Can you work these out from the model? Positions are in its coordinate system, mm. A direction names the side the tool comes from. Coordinates: 2 decimals unless noted, no trailing zeros. Write each loop counter-clockwise with the first axis right and the second up, starting at its lowest first coordinate (ties: lowest second). Pieces come first, ordered by that corner, then holes. Notation, with made-up numbers: (-37, 75) -> (-33, 75) arc R35 ccw to (-33, 108) -> close; hole circle Ø7 at (-14, -21). An arc over 180 degrees is marked (long way). Use one line per item in the form item = value.
```python
from build123d import *

# Parameters (mm, degrees)
SKETCH1_R           = 1.5
SKETCH1_W           = 4.5
SKETCH1_H           = 4.5
BOSS_EXTRUDE1_DEPTH = 2.5


with BuildPart() as part:
    # Sketch1 → Boss-Extrude1 (new body, symmetric)
    with BuildSketch(Plane(origin=(0, 0, 0), x_dir=(1, 0, 0), z_dir=(0, 1, 0))):
        with BuildLine():
            Line((-30, 50), (30, 50))
            ThreePointArc((30, 50), (33.535533906, 48.535533906), (35, 45))
            Line((35, 45), (35, -45))
            ThreePointArc((35, -45), (33.535533906, -48.535533906), (30, -50))
            Line((30, -50), (-30, -50))
            ThreePointArc((-30, -50), (-33.535533906, -48.535533906), (-35, -45))
            Line((-35, -45), (-35, 45))
            ThreePointArc((-35, 45), (-33.535533906, 48.535533906), (-30, 50))
        make_face()
        with Locations((10, 42)):
            Circle(SKETCH1_R, mode=Mode.SUBTRACT)
        with Locations((10, -42)):
            Circle(SKETCH1_R, mode=Mode.SUBTRACT)
        with Locations((-10, -42)):
            Circle(SKETCH1_R, mode=Mode.SUBTRACT)
        with Locations((-10, 42)):
            Circle(SKETCH1_R, mode=Mode.SUBTRACT)
        with Locations((28.5, 10)):
            Circle(SKETCH1_R, mode=Mode.SUBTRACT)
        with Locations((28.5, -10)):
            Circle(SKETCH1_R, mode=Mode.SUBTRACT)
        with Locations((-28.5, -10)):
            Circle(SKETCH1_R, mode=Mode.SUBTRACT)
        with Locations((-28.5, 10)):
            Circle(SKETCH1_R, mode=Mode.SUBTRACT)
        with Locations((27.25, 0)):
            Rectangle(SKETCH1_W, SKETCH1_H, mode=Mode.SUBTRACT)
        with Locations((0, -42.25)):
            Rectangle(SKETCH1_W, SKETCH1_H, mode=Mode.SUBTRACT)
        with Locations((0, 42.25)):
            Rectangle(SKETCH1_W, SKETCH1_H, mode=Mode.SUBTRACT)
        with Locations((-27.25, 0)):
            Rectangle(SKETCH1_W, SKETCH1_H, mode=Mode.SUBTRACT)
        with Locations((27.75, -42.75)):
            Rectangle(SKETCH1_W, SKETCH1_H, mode=Mode.SUBTRACT)
        with Locations((27.75, 42.75)):
            Rectangle(SKETCH1_W, SKETCH1_H, mode=Mode.SUBTRACT)
        with Locations((-27.75, 42.75)):
            Rectangle(SKETCH1_W, SKETCH1_H, mode=Mode.SUBTRACT)
        with Locations((-27.75, -42.75)):
            Rectangle(SKETCH1_W, SKETCH1_H, mode=Mode.SUBTRACT)
    extrude(amount=BOSS_EXTRUDE1_DEPTH, both=True)


solid = part.part
```
Q1. Suppose I cut it at B-B (x = -10). Write out the boundary of the cut face in (y, z), then the cut area to 3 significant figures.
Return value:
outline = (-2.5, -50) -> (2.5, -50) -> (2.5, -43.5) -> (-2.5, -43.5) -> close; (-2.5, -40.5) -> (2.5, -40.5) -> (2.5, 40.5) -> (-2.5, 40.5) -> close; (-2.5, 43.5) -> (2.5, 43.5) -> (2.5, 50) -> (-2.5, 50) -> close
area = 470 mm2
Q2. Thinking about a two-plate mould opening in Z: for faces 1 (the cylindrical face through (-10.325, -0.035, 43.464)), 2 (the flat face through (-35, 0, 1)), 3 (the cylindrical face through (-34, 0, -48)), which applies, released by +Z, released by -Z, zero draft, split by the parting line, or undercut?
Return value:
face_1 = undercut
face_2 = zero draft
face_3 = released by -Z
Q3. Will these pins go through, and if not, where does the flat tip stop? pin 1 (2.5 mm diameter, centred on x = -28.5, z = 10, fed in from +Y); pin 2 (3.5 mm diameter, centred on x = 28.5, z = 10, fed in from -Y).
Return value:
pin_1 = through
pin_2 = -2.5
Q4. Suppose I cut it at D-D (x = -28.5). Write out the boundary of the cut face in (y, z).
Return value:
outline = (-2.5, -50) -> (2.5, -50) -> (2.5, -45) -> (-2.5, -45) -> close; (-2.5, -40.5) -> (2.5, -40.5) -> (2.5, -11.5) -> (-2.5, -11.5) -> close; (-2.5, -8.5) -> (2.5, -8.5) -> (2.5, -2.25) -> (-2.5, -2.25) -> close; (-2.5, 2.25) -> (2.5, 2.25) -> (2.5, 8.5) -> (-2.5, 8.5) -> close; (-2.5, 11.5) -> (2.5, 11.5) -> (2.5, 40.5) -> (-2.5, 40.5) -> close; (-2.5, 45) -> (2.5, 45) -> (2.5, 50) -> (-2.5, 50) -> close
Q5. Suppose I cut it at A-A (z = 42). Write out the boundary of the cut face in (x, y).
Return value:
outline = (-35, -2.5) -> (-30, -2.5) -> (-30, 2.5) -> (-35, 2.5) -> close; (-25.5, -2.5) -> (-11.5, -2.5) -> (-11.5, 2.5) -> (-25.5, 2.5) -> close; (-8.5, -2.5) -> (-2.25, -2.5) -> (-2.25, 2.5) -> (-8.5, 2.5) -> close; (2.25, -2.5) -> (8.5, -2.5) -> (8.5, 2.5) -> (2.25, 2.5) -> close; (11.5, -2.5) -> (25.5, -2.5) -> (25.5, 2.5) -> (11.5, 2.5) -> close; (30, -2.5) -> (35, -2.5) -> (35, 2.5) -> (30, 2.5) -> close
Q6. If I drill on line 1 (Z direction, x = -10, y = -1.4); line 2 (X direction, y = 1.35, z = 10); line 3 (Z direction, x = -28.5, y = 1.1), over which ranges is the centre line in solid material (lowest first)? Write a range as from..to.
Return value:
line_1 = -50..-43.5, -40.5..40.5, 43.5..50
line_2 = -35..-30, -27..27, 30..35
line_3 = -50..-45, -40.5..-11.5, -8.5..-2.25, 2.25..8.5, 11.5..40.5, 45..50
Q7. For faces 4 (the flat face through (30, 0, 43)), 5 (the cylindrical face through (33, 0, -49)), which set-ups out of +Z, -Z, +X, -X, +Y, -Y let a thin tool reach every point of the face, with its end or its side?
Return value:
face_4 = +Y, -Y
face_5 = -Z, +X, +Y, -Y
Q8. Suppose I cut it at C-C (z = 0). Write out the boundary of the cut face in (x, y), then the cut area to 3 significant figures.
Return value:
outline = (-35, -2.5) -> (-29.5, -2.5) -> (-29.5, 2.5) -> (-35, 2.5) -> close; (-25, -2.5) -> (25, -2.5) -> (25, 2.5) -> (-25, 2.5) -> close; (29.5, -2.5) -> (35, -2.5) -> (35, 2.5) -> (29.5, 2.5) -> close
area = 305 mm2
